```python
from build123d import *

# Parameters (mm, degrees)
F0_W     = 20
F0_H     = 20
F0_R     = 5.5
F1_DEPTH = 20
F5_R     = 7.5
F6_DEPTH = 10


with BuildPart() as f1:
    # F0 (on Front) → F1 (new body)
    with BuildSketch(Plane.XZ):
        with Locations((-10, 10)):
            Rectangle(F0_W, F0_H)
        with Locations((-10, 10)):
            Circle(F0_R, mode=Mode.SUBTRACT)
    extrude(amount=-F1_DEPTH)

    # F3 (on offset) → F4 (revolve, cut)
    with BuildSketch(Plane.YZ.offset(-10)):
        with BuildLine():
            ThreePointArc((0, 16), (0.7791287847, 16.5), (0, 17))
            Line((0, 17), (0, 16))
        make_face()
    revolve(axis=Axis((-10, 6.498338189, 10), (0, 1, 0)), mode=Mode.SUBTRACT)

    # F5 (on face) → F6 (cut)
    with BuildSketch(Plane(origin=(0, 20, 0), x_dir=(-1, 0, 0), z_dir=(0, 1, 0))):
        with Locations((10, 10)):
            Circle(F5_R)
    extrude(amount=-F6_DEPTH, mode=Mode.SUBTRACT)


solid = f1.part
```
CAD build for the part. Positions are in the model's coordinates, mm. A direction names the side the tool comes from. Coordinates: 2 decimals unless noted, no trailing zeros. Loops run counter-clockwise (first coordinate to the right, second up) from the corner with the lowest first, then second, coordinate; pieces in that order, holes last. Notation, with made-up numbers: (63, 53) - (103, 53) arc R19 ccw to (103, 59) - close; hole circle Ø7 at (1, 22.25). An arc over 180 degrees is marked (long way). Return JSON: item names as keys, results as strings.
1. Mould opens along Z. For faces 3 (the cylindrical face through (-8.37, 15.07, 2.68)), 4 (the flat face through (-10, 10, 0)), 5 (the flat face through (-17, 0, 12)) say: released by +Z, released by -Z, zero draft, split by the parting line, or undercut.
Result:
{"face 3": "undercut", "face 4": "released by -Z", "face 5": "zero draft"}
2. 3-axis set-ups, long thin cutter, end or side, ignore diameter. For faces 1 (the flat face through (-20, 10, 10)), 2 (the flat face through (-6, 10, 14)): which of +Z, -Z, +X, -X, +Y, -Y reach the whole face in a straight line?
Result:
{"face 1": "+Z, -Z, -X, +Y, -Y", "face 2": "+Y"}
3. Band-saw the part on B-B (y = 6.75). Give the cut face in (x, z).
Result:
{"outline": "(-20, 0) - (0, 0) - (0, 20) - (-20, 20) - close; hole circle Ø11 at (-10, 10)"}
4. Band-saw the part on D-D (y = 15.75). Give the cut face in (x, z).
Result:
{"outline": "(-20, 0) - (0, 0) - (0, 20) - (-20, 20) - close; hole circle Ø15 at (-10, 10)"}
5. Drop a flat-ended pin along its axis: pin 1 (6.5 mm diameter, centred on x = -10, z = 10, fed in from +Y). Give the stop position or say it passes through.
Result:
{"pin 1": "passes through"}
6. Band-saw the part on A-A (x = -10). Give the cut face in (y, z), and give its area (3 significant figures).
Result:
{"outline": "(0, 0) - (20, 0) - (20, 2.5) - (10, 2.5) - (10, 4.5) - (0, 4.5) - (0, 4) arc R0.55 cw (long way) to (0, 3) - close; (0, 15.5) - (10, 15.5) - (10, 17.5) - (20, 17.5) - (20, 20) - (0, 20) - (0, 17) arc R0.55 cw (long way) to (0, 16) - close", "area": "139 mm2"}
7. Band-saw the part on C-C (z = 10). Give the cut face in (x, y), and give its area (3 significant figures).
Result:
{"outline": "(-20, 0) - (-17, 0) arc R0.55 cw (long way) to (-16, 0) - (-15.5, 0) - (-15.5, 10) - (-17.5, 10) - (-17.5, 20) - (-20, 20) - close; (-4.5, 0) - (-4, 0) arc R0.55 cw (long way) to (-3, 0) - (0, 0) - (0, 20) - (-2.5, 20) - (-2.5, 10) - (-4.5, 10) - close", "area": "139 mm2"}
8. Probe L1, parallel to Z at x = -10, y = 12.75; L2, parallel to Z at x = -10, y = 3.5; L3, parallel to Y at x = -4, z = 6. List the from-to ranges inside material, lowest first. Write a range as from..to.
Result:
{"L1": "z = 0..2.5, 17.5..20", "L2": "z = 0..4.5, 15.5..20", "L3": "y = 0..10"}
